Part model, mm, in its own coordinate system. A direction names the side the tool comes from. Round coordinates to 2 decimals unless told otherwise and drop trailing zeros. Order: outer loops, then holes, each group sorted by start corner. A loop starts at its lowest first (then second) coordinate and runs counter-clockwise, first axis right, second up. Notation, with made-up numbers: M 60,-25.75 L 92,-25.75 A19 ccw 92,6.25 Z; hole C 21,-21.5 d6. An arc over 180 degrees is marked long. One line per question, with ' | ' between items.
from build123d import *

# Parameters (mm, degrees)
SKETCH1_W           = 75
SKETCH1_H           = 60
BOSS_EXTRUDE1_DEPTH = 24
SKETCH2_R           = 2
CUT_EXTRUDE1_DEPTH  = 25
SKETCH3_W           = 45
SKETCH3_H           = 40
CUT_EXTRUDE2_DEPTH  = 15
SKETCH4_R           = 5
CUT_EXTRUDE3_DEPTH  = 11
SKETCH5_R           = 5.9
CUT_EXTRUDE4_DEPTH  = 10


with BuildPart() as part:
    # Sketch1 → Boss-Extrude1 (new body)
    with BuildSketch(Plane(origin=(0, 0, 0), x_dir=(1, 0, 0), z_dir=(0, 1, 0))):
        with Locations((37.5, 30)):
            Rectangle(SKETCH1_W, SKETCH1_H)
    extrude(amount=BOSS_EXTRUDE1_DEPTH)

    # Sketch2 → Cut-Extrude1 (cut, through all)
    with BuildSketch(Plane(origin=(0, 24, 0), x_dir=(1, 0, 0), z_dir=(0, 1, 0))):
        with Locations((6, 54)):
            Circle(SKETCH2_R)
        with Locations((6, 6)):
            Circle(SKETCH2_R)
        with Locations((69, 54)):
            Circle(SKETCH2_R)
        with Locations((69, 6)):
            Circle(SKETCH2_R)
    extrude(amount=-CUT_EXTRUDE1_DEPTH, mode=Mode.SUBTRACT)

    # Sketch3 → Cut-Extrude2 (cut)
    with BuildSketch(Plane.XZ):
        with Locations((37.5, -30)):
            Rectangle(SKETCH3_W, SKETCH3_H)
    extrude(amount=-CUT_EXTRUDE2_DEPTH, mode=Mode.SUBTRACT)

    # Sketch4 → Cut-Extrude3 (cut, through all)
    with BuildSketch(Plane(origin=(0, 0, -10), x_dir=(-1, 0, 0), z_dir=(0, 0, -1))):
        with Locations((-21, 10)):
            Circle(SKETCH4_R)
    extrude(amount=-CUT_EXTRUDE3_DEPTH, mode=Mode.SUBTRACT)

    # Sketch5 → Cut-Extrude4 (cut)
    with BuildSketch(Plane.XY):
        with Locations((21, 10)):
            Circle(SKETCH5_R)
    extrude(amount=-CUT_EXTRUDE4_DEPTH, mode=Mode.SUBTRACT)


solid = part.part
1) Saw through at D-D (z = -54). List the corners of the cut face in (x, y).
The answers:
outline: M 0,0 L 4,0 L 4,24 L 0,24 Z; M 8,0 L 67,0 L 67,24 L 8,24 Z; M 71,0 L 75,0 L 75,24 L 71,24 Z
2) Saw through at C-C (y = 10). List the corners of the cut face in (x, z), plus the area to 3 significant figures.
The answers:
outline: M 0,-60 L 75,-60 L 75,0 L 26.9,0 L 26.9,-10 L 60,-10 L 60,-50 L 15,-50 L 15,-10 L 15.1,-10 L 15.1,0 L 0,0 Z; hole C 6,-54 d4; hole C 6,-6 d4; hole C 69,-54 d4; hole C 69,-6 d4 | area: 2,530 mm²
3) Drop flat-ended pins along their axis: pin 1 (3.5 mm diameter, centred on x = 6, z = -54, fed in from +Y); pin 2 (8 mm diameter, centred on x = 20.5, z = -38.5, fed in from -Y); pin 3 (0.7 mm diameter, centred on x = 21, y = 15.5, fed in from +Z). Give the stop position or say it passes through.
The answers:
pin 1: passes through | pin 2: stops at y = 15 | pin 3: stops at z = -10
4) Probe line 1 (Z direction, x = 6, y = 9.25); line 2 (X direction, y = 10.75, z = -54); line 3 (X direction, y = 11.5, z = -40). List the from-to ranges inside material, lowest first. Write a range as [from, to].
The answers:
line 1: z = [-60, -56], [-52, -8], [-4, 0] | line 2: x = [0, 4], [8, 67], [71, 75] | line 3: x = [0, 15], [60, 75]
5) Two-plate mould, pull along Z, no slides. Class faces 4 (the face through (42, 7, -10)), 5 (the face through (0, 12, -30)), 6 (the face through (4.526, 12.168, -7.352)), 7 (the face through (37, 12, 0)): released by +Z, released by -Z, zero draft, split by the parting line, or undercut.
The answers:
face 4: undercut | face 5: zero draft | face 6: undercut | face 7: released by +Z
6) Saw through at A-A (x = 6). List the corners of the cut face in (y, z), plus the area to 3 significant figures.
The answers:
outline: M 0,-60 L 24,-60 L 24,-56 L 0,-56 Z; M 0,-52 L 24,-52 L 24,-8 L 0,-8 Z; M 0,-4 L 24,-4 L 24,0 L 0,0 Z | area: 1,250 mm²
7) Saw through at B-B (z = -6). List the corners of the cut face in (x, y).
The answers:
outline: M 0,0 L 4,0 L 4,24 L 0,24 Z; M 8,0 L 67,0 L 67,24 L 8,24 Z; M 71,0 L 75,0 L 75,24 L 71,24 Z; hole C 21,10 d11.8
8) Which spindle directions (+Z, -Z, +X, -X, +Y, -Y) get a long thin tool onto all of the face, cutting with end or side? Do faces 1 (the face through (15.106, 10.259, -4.93)), 2 (the face through (60, 7, -30)), 3 (the face through (75, 12, -30)). Say none if no direction does.
The answers:
face 1: +Z | face 2: -Y | face 3: +Z, -Z, +X, +Y, -Y
